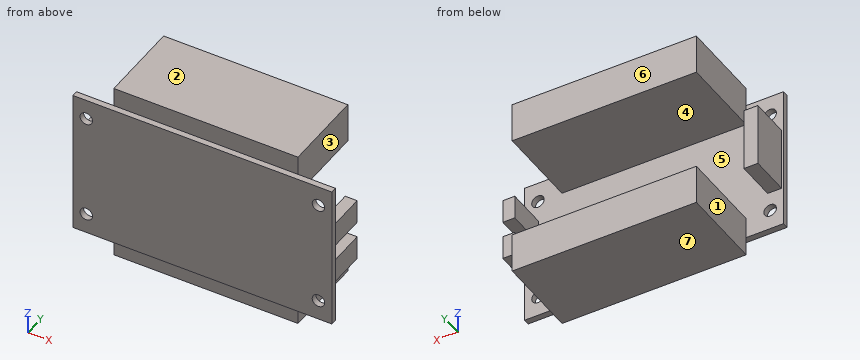
from build123d import *

# Parameters (mm, degrees)
SKETCH1_W           = 65.03
SKETCH1_H           = 36.54
SKETCH1_R           = 1.57
BOSS_EXTRUDE1_DEPTH = 1.5
SKETCH2_W           = 3
SKETCH2_H           = 6
SKETCH2_W_2         = 3.5
SKETCH2_H_2         = 16
BOSS_EXTRUDE2_DEPTH = 10
SKETCH3_W           = 46.23
SKETCH3_H           = 10
BOSS_EXTRUDE3_DEPTH = 21


with BuildPart() as part:
    # Sketch1 → Boss-Extrude1 (new body)
    with BuildSketch(Plane(origin=(0, 0, 0), x_dir=(1, 0, 0), z_dir=(0, 1, 0))):
        Rectangle(SKETCH1_W, SKETCH1_H)
        with Locations(Location((-29.145, 13.2, 0), (0, 0, 270))):
            Circle(SKETCH1_R, mode=Mode.SUBTRACT)
        with Locations(Location((29.145, 13.2, 0), (0, 0, 90))):
            Circle(SKETCH1_R, mode=Mode.SUBTRACT)
        with Locations(Location((29.145, -13.2, 0), (0, 0, 270))):
            Circle(SKETCH1_R, mode=Mode.SUBTRACT)
        with Locations(Location((-29.145, -13.2, 0), (0, 0, 90))):
            Circle(SKETCH1_R, mode=Mode.SUBTRACT)
    extrude(amount=BOSS_EXTRUDE1_DEPTH)

    # Sketch2 → Boss-Extrude2 (add)
    with BuildSketch(Plane(origin=(0, 1.5, 0), x_dir=(1, 0, 0), z_dir=(0, 1, 0))):
        with Locations((30.515, -4.73)):
            Rectangle(SKETCH2_W, SKETCH2_H)
        with Locations((-30.265, 0.27)):
            Rectangle(SKETCH2_W_2, SKETCH2_H_2)
        with Locations((30.515, 5.27)):
            Rectangle(SKETCH2_W, SKETCH2_H)
    extrude(amount=BOSS_EXTRUDE2_DEPTH)

    # Sketch3 → Boss-Extrude3 (add)
    with BuildSketch(Plane(origin=(0, 1.5, 0), x_dir=(1, 0, 0), z_dir=(0, 1, 0))):
        with Locations((0, -18.030936004)):
            Rectangle(SKETCH3_W, SKETCH3_H)
        with Locations((0, 18.030936004)):
            Rectangle(SKETCH3_W, SKETCH3_H)
    extrude(amount=BOSS_EXTRUDE3_DEPTH)


solid = part.part
Design review of the part built by this model. Coordinates are the model's own, in mm. Face numbers are marked on the shaded views. A direction names the side the tool comes from. Coordinates: 2 decimals unless noted, no trailing zeros. Order: outer loops, then holes, each group sorted by start corner. A loop starts at its lowest first (then second) coordinate and runs counter-clockwise, first axis right, second up. Notation, with made-up numbers: (-38, -37) -> (-23, -37) arc R18 cw to (-23, -20) -> close; hole circle Ø4 at (-33.75, 67.25). An arc over 180 degrees is marked (long way). One line per item, written item: value.
1) We need section B-B, the plane y = 20.75. Give the boundary of the cut face in (x, z) (3 decimals).
Output values:
outline: (-23.115, -23.031) -> (23.115, -23.031) -> (23.115, -13.031) -> (-23.115, -13.031) -> close; (-23.115, 13.031) -> (23.115, 13.031) -> (23.115, 23.031) -> (-23.115, 23.031) -> close
2) Machinability: for the marked faces 1, 2 and 3, which of the approach directions +Z, -Z, +X, -X, +Y, -Y give a long, thin tool a straight path to every point of the face, cutting with its end or side? Answer none if there is none.
Output values:
face 1: +Z, -Z, -X, +Y
face 2: +Z, +X, -X, +Y, -Y
face 3: +Z, -Z, +X, +Y
3) Clearance check with flat-ended pins moving along their axes: P1, Ø1.2, axis at x = 11.5, y = 0.5, coming from the +Z side; P2, Ø11, axis at x = 3, z = -9, coming from the +Y side; P3, Ø3, axis at y = 4.5, z = -2, coming from the +X side (3 decimals); P4, Ø0.9, axis at x = 30.5, y = 5.5, coming from the -Z side. State where each tip first meets the part, or that it passes through.
Output values:
P1: stops at z = 18.27
P2: stops at y = 22.5
P3: stops at x = 32.015
P4: stops at z = -8.27
4) To check wall thickness, follow probe 1 along X at (y, z) = (0.8, 13.2) (3 decimals); probe 2 along Z at (x, y) = (12, 16.5); probe 3 along Y at (x, z) = (-17, 12). State the ranges of each line that lie inside material, in increasing order. Write a range as [from, to].
Output values:
probe 1: x = [-32.515, -30.715], [-27.575, 27.575], [30.715, 32.515]
probe 2: z = [-23.03, -13.03], [13.03, 23.03]
probe 3: y = [0, 1.5]
5) We need section C-C, the plane z = -5.5. Give the boundary of the cut face in (x, y) (3 decimals), then the cut area to 3 significant figures.
Output values:
outline: (-32.515, 0) -> (32.515, 0) -> (32.515, 1.5) -> (32.015, 1.5) -> (32.015, 11.5) -> (29.015, 11.5) -> (29.015, 1.5) -> (-28.515, 1.5) -> (-28.515, 11.5) -> (-32.015, 11.5) -> (-32.015, 1.5) -> (-32.515, 1.5) -> close
area: 163 mm2
6) Draft analysis for pull direction Z (two halves, no side actions). For the marked faces 4, 5, 6 and 7, state which applies: +Z half, -Z half, draft (parallel to the pull), parting line (faces both ways), or undercut.
Output values:
face 4: undercut
face 5: undercut
face 6: draft
face 7: -Z half
7) We need section D-D, the plane x = -21.5. Give the boundary of the cut face in (y, z), then the cut area to 3 significant figures.
Output values:
outline: (0, -18.27) -> (1.5, -18.27) -> (1.5, -23.03) -> (22.5, -23.03) -> (22.5, -13.03) -> (1.5, -13.03) -> (1.5, 13.03) -> (22.5, 13.03) -> (22.5, 23.03) -> (1.5, 23.03) -> (1.5, 18.27) -> (0, 18.27) -> close
area: 475 mm2
8) We need section A-A, the plane y = 10. Give the boundary of the cut face in (x, z) (3 decimals), then the cut area to 3 significant figures.
Output values:
outline: (-32.015, -8.27) -> (-28.515, -8.27) -> (-28.515, 7.73) -> (-32.015, 7.73) -> close; (-23.115, -23.031) -> (23.115, -23.031) -> (23.115, -13.031) -> (-23.115, -13.031) -> close; (-23.115, 13.031) -> (23.115, 13.031) -> (23.115, 23.031) -> (-23.115, 23.031) -> close; (29.015, -8.27) -> (32.015, -8.27) -> (32.015, -2.27) -> (29.015, -2.27) -> close; (29.015, 1.73) -> (32.015, 1.73) -> (32.015, 7.73) -> (29.015, 7.73) -> close
area: 1,020 mm2
